The listing builds one solid part. Answer for the finished solid, in the listing's coordinates (mm). A direction names the side the tool comes from. Coordinates: 2 decimals unless noted, no trailing zeros. Write each loop counter-clockwise with the first axis right and the second up, starting at its lowest first coordinate (ties: lowest second). Pieces come first, ordered by that corner, then holes.
(1) Given P1, Ø1.9, axis at x = 3.25, y = 50.5, coming from the -Z side; P2, Ø6, axis at x = 24, y = 43, coming from the +Z side; P3, Ø0.9, axis at x = 25.5, z = 1.5, coming from the +Y side, each flat-ended and moving along its own axis, determine where each tip first touches the part or whether it passes through.
(2) The part is cut by section B-B on x = 33.75. Determine the outline of the cut face in (y, z), plus the area to 3 significant figures.
(3) Straight lines are drawn through the part: line 1 (Y direction, x = 3.25, z = -0.8); line 2 (X direction, y = 64, z = 2.3); line 3 (Z direction, x = 8, y = 4). For each, find the intervals that lie inside material, in ascending order.
(4) The part is cut by section D-D on x = 11. Determine the outline of the cut face in (y, z), plus the area to 3 significant figures.
(5) The part is cut by section C-C on y = 50.5. Determine the outline of the cut face in (x, z), plus the area to 3 significant figures.
(6) Which of the six approach directions +Z, -Z, +X, -X, +Y, -Y give full straight-line access (tool end or side, diameter ignored) to faces 1 (the flat face through (38, 60.25, 2)), 2 (the flat face through (38, 67, 3)), 3 (the flat face through (37, 5, 1))?
(7) For a pull along Y with two mould halves and no side action, classify faces 4 (the flat face through (19, -2.5, 0)), 5 (the flat face through (18, 0, 1)), 6 (the flat face through (19, -1, 3)), 7 (the flat face through (38, 10.25, 2)) as +Y half, -Y half, draft (parallel to the pull), parting line (faces both ways), or undercut.
(8) The part is cut by section A-A on z = 2.25. Determine the outline of the cut face in (x, y).
from build123d import *

# Parameters (mm, degrees)
EXTRUDE_THIN1_DEPTH        = 3
SKETCH2_W                  = 42
SKETCH2_H                  = 75.5
BOSS_EXTRUDE2_DEPTH        = 3
F_3_2_3_2_DIAMETER_HOLE1_D = 3.2
SKETCH6_W                  = 2.5
SKETCH6_H                  = 50
CUT_EXTRUDE1_DEPTH         = 3


with BuildPart() as part:
    # Sketch1 → Extrude-Thin1 (new body)
    with BuildSketch(Plane.XY):
        Polygon((0, 73), (0, 0), (37, 0), (37, 73), (39.5, 73), (39.5, -2.5), (-2.5, -2.5), (-2.5, 73), align=None)
    extrude(amount=EXTRUDE_THIN1_DEPTH)

    # Sketch2 → Boss-Extrude2 (add)
    with BuildSketch(Plane(origin=(0, 0, 0), x_dir=(-1, 0, 0), z_dir=(0, 0, -1))):
        with Locations((-18.5, 35.25)):
            Rectangle(SKETCH2_W, SKETCH2_H)
    extrude(amount=BOSS_EXTRUDE2_DEPTH)

    # Ø3.2 (3.2) Diameter Hole1 (through all)
    with Locations(Plane.XY):
        with Locations((3.25, 50.5), (33.75, 50.5), (33.75, 20), (3.25, 20)):
            Hole(F_3_2_3_2_DIAMETER_HOLE1_D / 2)

    # Sketch6 → Cut-Extrude1 (cut)
    with BuildSketch(Plane.XY.offset(3)):
        with Locations((-1.25, 35.25)):
            Rectangle(SKETCH6_W, SKETCH6_H)
    cut_extrude1 = extrude(amount=-CUT_EXTRUDE1_DEPTH, mode=Mode.SUBTRACT)

    # Mirror1: Cut-Extrude1 across plane
    add(cut_extrude1.mirror(Plane(origin=(18.5, 0, 0), x_dir=(0, 0, 1), z_dir=(1, 0, 0))), mode=Mode.SUBTRACT)


solid = part.part
Model answer:
1. P1: passes through
1. P2: stops at z = 0
1. P3: stops at y = 0
2. outline: (-2.5, -3) - (18.4, -3) - (18.4, 0) - (0, 0) - (0, 3) - (-2.5, 3) - close; (21.6, -3) - (48.9, -3) - (48.9, 0) - (21.6, 0) - close; (52.1, -3) - (73, -3) - (73, 0) - (52.1, 0) - close
2. area: 215 mm2
3. line 1: y = -2.5 to 18.4, 21.6 to 48.9, 52.1 to 73
3. line 2: x = -2.5 to 0, 37 to 39.5
3. line 3: z = -3 to 0
4. outline: (-2.5, -3) - (73, -3) - (73, 0) - (0, 0) - (0, 3) - (-2.5, 3) - close
4. area: 234 mm2
5. outline: (-2.5, -3) - (1.65, -3) - (1.65, 0) - (-2.5, 0) - close; (4.85, -3) - (32.15, -3) - (32.15, 0) - (4.85, 0) - close; (35.35, -3) - (39.5, -3) - (39.5, 0) - (35.35, 0) - close
5. area: 107 mm2
6. face 1: +Z, +X, -X
6. face 2: +Z, +X, -X, +Y, -Y
6. face 3: +Z, +Y
7. face 4: -Y half
7. face 5: +Y half
7. face 6: draft
7. face 7: undercut
8. outline: (-2.5, -2.5) - (39.5, -2.5) - (39.5, 10.25) - (37, 10.25) - (37, 0) - (0, 0) - (0, 10.25) - (-2.5, 10.25) - close; (-2.5, 60.25) - (0, 60.25) - (0, 73) - (-2.5, 73) - close; (37, 60.25) - (39.5, 60.25) - (39.5, 73) - (37, 73) - close
